Could you check a few things on this model? Use its own coordinates, in mm. A direction names the side the tool comes from. Coordinates: 2 decimals unless noted, no trailing zeros. Loops run counter-clockwise (first coordinate to the right, second up) from the corner with the lowest first, then second, coordinate; pieces in that order, holes last.
1) If I drill on line 1 along X through (y, z) = (1.2, 0); line 2 along Y through (x, z) = (-1.5, -5); line 3 along X through (y, z) = (13.75, 1.5), over which ranges is the centre line in solid material (lowest first)?
2) Thinking about a two-plate mould opening in X: for faces 4 (the face through (17.696, 2.535, 9.289)), 5 (the face through (-9.87, 2.15, -0.28)), 6 (the face through (0, 27, -5)), which applies, released by +X, released by -X, zero draft, split by the parting line, or undercut?
3) Imagine slicing it at B-B on z = 0. Please give me the cut outline in (x, y), plus the area to 3 significant figures.
4) Imagine slicing it at A-A on x = -12. Please give me the cut outline in (y, z).
5) For faces 1 (the face through (-5, 16, 3)), 2 (the face through (0, 22, -8)), 3 (the face through (5, 16, 3)), which set-ups out of +Z, -Z, +X, -X, +Y, -Y let a thin tool reach every point of the face, with its end or its side?
6) Will these pins go through, and if not, where does the flat tip stop? P1, Ø3, axis at y = 15.5, z = 6.5, coming from the +X side; P2, Ø11, axis at y = 18, z = -2, coming from the -X side; P3, Ø7, axis at x = 15, z = -4, coming from the +Y side; P4, Ø3, axis at x = 12, z = 0, coming from the +Y side.
7) Imagine slicing it at D-D on z = -6.5. Please give me the cut outline in (x, y), plus the area to 3 significant figures.
```python
from build123d import *

# Parameters (mm, degrees)
SKETCH1_W           = 39
SKETCH1_H           = 22
BOSS_EXTRUDE1_DEPTH = 5
SKETCH2_W           = 10
SKETCH2_H           = 22
BOSS_EXTRUDE2_DEPTH = 22
SKETCH3_W           = 10
SKETCH3_H           = 12.5
CUT_EXTRUDE1_DEPTH  = 12.5
FILLET1_R           = 6.25
FILLET2_R           = 6
FILLET3_R           = 9
SKETCH5_R           = 2
CUT_EXTRUDE3_DEPTH  = 32.388692231
FILLET4_R           = 6
CHAMFER4_SIZE       = 3


# Some blends are built 0.0001 mm under size
with BuildPart() as part:
    # Sketch1 → Boss-Extrude1 (new body)
    with BuildSketch(Plane(origin=(0, 0, 0), x_dir=(1, 0, 0), z_dir=(0, 1, 0))):
        Rectangle(SKETCH1_W, SKETCH1_H)
    extrude(amount=BOSS_EXTRUDE1_DEPTH)

    # Sketch2 → Boss-Extrude2 (add)
    with BuildSketch(Plane(origin=(0, 5, 0), x_dir=(1, 0, 0), z_dir=(0, 1, 0))):
        Rectangle(SKETCH2_W, SKETCH2_H)
    extrude(amount=BOSS_EXTRUDE2_DEPTH)

    # Sketch3 → Cut-Extrude1 (cut)
    with BuildSketch(Plane(origin=(0, 0, -11), x_dir=(-1, 0, 0), z_dir=(0, 0, -1))):
        with Locations((0, 15.75)):
            Rectangle(SKETCH3_W, SKETCH3_H)
    extrude(amount=-CUT_EXTRUDE1_DEPTH, mode=Mode.SUBTRACT)

    # Fillet1
    fillet1_edges = [part.edges().sort_by_distance(p)[0] for p in [
        (0, 22, 1.5),
        (0, 9.5, 1.5),
    ]]
    fillet(fillet1_edges, radius=FILLET1_R - 0.0001)  # a hair under: the kernel refuses the full size

    # Fillet2
    fillet2_edges = [part.edges().sort_by_distance(p)[0] for p in [
        (-19.5, 2.5, -11),
        (19.5, 2.5, -11),
        (19.5, 2.5, 11),
        (-19.5, 2.5, 11),
    ]]
    fillet(fillet2_edges, radius=FILLET2_R)

    # Fillet3
    fillet3_edges = [part.edges().sort_by_distance(p)[0] for p in [
        (0, 27, 11),
    ]]
    fillet(fillet3_edges, radius=FILLET3_R)

    # Sketch5 → Cut-Extrude3 (cut, through all)
    with BuildSketch(Plane(origin=(0, 5, 0), x_dir=(1, 0, 0), z_dir=(0, 1, 0))):
        with Locations(Location((-12, 0, 0), (0, 0, 270))):
            Circle(SKETCH5_R)
        with Locations(Location((12, 0, 0), (0, 0, 270))):
            Circle(SKETCH5_R)
    extrude(amount=-CUT_EXTRUDE3_DEPTH, mode=Mode.SUBTRACT)

    # Fillet4
    # the kernel refuses this fillet: 6 mm, written as the material it takes off along each edge
    with BuildSketch(Plane(origin=(-20, 9.5, -11), x_dir=(0, -1, 0), z_dir=(1, 0, 0))) as fillet4_piece_1:
        with BuildLine():
            CenterArc((FILLET4_R, -FILLET4_R), FILLET4_R, 90, 90)
            Line((0, -FILLET4_R), (0, 0))
            Line((0, 0), (FILLET4_R, 0))
        make_face()
    extrude(amount=40, mode=Mode.SUBTRACT)

    # Chamfer4
    chamfer4_edges = [part.edges().sort_by_distance(p)[0] for p in [
        (-12, 5, -2),
        (12, 5, -2),
    ]]
    chamfer(chamfer4_edges, length=CHAMFER4_SIZE)


solid = part.part
```
Filled in:
1. line 1: x = -19.5 to -14, -10 to 10, 14 to 19.5
1. line 2: y = 0 to 9.5, 22 to 27
1. line 3: x = -5 to 5
2. face 4: released by +X
2. face 5: undercut
2. face 6: zero draft
3. outline: (-19.5, 0) - (-14, 0) - (-14, 2) - (-17, 5) - (-19.5, 5) - close; (-10, 0) - (10, 0) - (10, 2) - (7, 5) - (5, 5) - (5, 11.69) - (-5, 11.69) - (-5, 5) - (-7, 5) - (-10, 2) - close; (-5, 19.81) - (5, 19.81) - (5, 27) - (-5, 27) - close; (14, 0) - (19.5, 0) - (19.5, 5) - (17, 5) - (14, 2) - close
3. area: 276 mm2
4. outline: (0, -11) - (3.5, -11) arc R6 ccw to (5, -10.81) - (5, -5) - (2, -2) - (0, -2) - close; (0, 2) - (2, 2) - (5, 5) - (5, 11) - (0, 11) - close
5. face 1: +Z, -Z, -X, +Y
5. face 2: -Z, +X, -X
5. face 3: +Z, -Z, +X, +Y
6. P1: stops at x = 5
6. P2: stops at x = -5
6. P3: stops at y = 5
6. P4: passes through
7. outline: (-19.31, 0) - (19.31, 0) - (19.31, 5) - (5, 5) - (5, 9.31) - (-5, 9.31) - (-5, 5) - (-19.31, 5) - close; (-5, 22) - (5, 22) - (5, 27) - (-5, 27) - close
7. area: 286 mm2
